Here's how the part is built. I have some questions about the finished solid (model axes, mm). Coordinates: 2 decimals unless noted, no trailing zeros. Write each loop counter-clockwise with the first axis right and the second up, starting at its lowest first coordinate (ties: lowest second). Pieces come first, ordered by that corner, then holes. Notation, with made-up numbers: (70, -27.5) - (123, -27.5) arc R15 ccw to (123, -12.5) - close; hole circle Ø5 at (59.25, 47). An arc over 180 degrees is marked (long way). Answer in a Markdown table with one row per item. Add a question column.
Item 1: If I drill on probe 1 along Z at (x, y) = (-12.5, 2.7) (3 decimals); probe 2 along Z at (x, y) = (24.6, 0.85) (3 decimals); probe 3 along Z at (x, y) = (-24.5, 1.9) (3 decimals), over which ranges is the centre line in solid material (lowest first)? Write a range as from..to.
Item 2: Imagine slicing it at A-A (x = 24.6). Please give me the cut outline in (y, z) (3 decimals).
Item 3: Imagine slicing it at C-C (x = 3.5). Please give me the cut outline in (y, z), plus the area to 3 significant figures.
Item 4: Imagine slicing it at D-D (z = 0). Please give me the cut outline in (x, y) (1 decimal).
Item 5: Imagine slicing it at B-B (z = 25.8). Please give me the cut outline in (x, y) (3 decimals), plus the area to 3 significant figures.
Autodesk Inventor part; units mm, degrees
ref_plane "YZ Plane" through (0, 0, 0) normal (1, 0, 0) x (0, 1, 0)
ref_plane "XZ Plane" through (0, 0, 0) normal (0, 1, 0) x (-1, 0, 0)
ref_plane "XY Plane" through (0, 0, 0) normal (0, 0, 1) x (1, 0, 0)
sketch "Boceto1" plane through (0, 0, 0) normal (0, 1, 0) x (-1, 0, 0)
  line L0 (-31.7268, 34.9358) -> (-31.7268, -34.7768)
  line L1 (-28.9268, -37.5768) -> (25.401, -37.5769)
  line L2 (28.2018, -34.7802) -> (28.2019, 34.9339)
  line L3 (25.4109, 37.7268) -> (-28.9358, 37.7268)
  line L4 (-29.925, -4.425) -> (-29.925, 4.575)
  line L5 (-29.925, 4.575) -> (-29.85, 4.575)
  line L6 (-29.85, 4.575) -> (-27.6, 4.575)
  line L7 (-27.6, 4.575) -> (-27.525, 4.575)
  line L8 (-27.525, 4.575) -> (-27.525, -4.425)
  line L9 (-27.525, -4.425) -> (-27.6, -4.425)
  line L10 (-27.6, -4.425) -> (-29.85, -4.425)
  line L11 (-29.85, -4.425) -> (-29.925, -4.425)
  line L12 (26.4, -4.425) -> (26.325, -4.425)
  line L13 (26.325, -4.425) -> (24.075, -4.425)
  line L14 (24.075, -4.425) -> (24, -4.425)
  line L15 (24, -4.425) -> (24, 4.575)
  line L16 (24, 4.575) -> (24.075, 4.575)
  line L17 (24.075, 4.575) -> (26.325, 4.575)
  line L18 (26.325, 4.575) -> (26.4, 4.575)
  line L19 (26.4, 4.575) -> (26.4, -4.425)
  line L20 (26.325, 26.925) -> (26.4, 26.925)
  line L21 (26.4, 26.925) -> (26.4, 17.925)
  line L22 (26.4, 17.925) -> (26.325, 17.925)
  line L23 (26.325, 17.925) -> (24.075, 17.925)
  line L24 (24.075, 17.925) -> (24, 17.925)
  line L25 (24, 17.925) -> (24, 26.925)
  line L26 (24, 26.925) -> (24.075, 26.925)
  line L27 (24.075, 26.925) -> (26.325, 26.925)
  line L28 (-19.1813, -35.775) -> (-19.1813, -35.7)
  line L29 (-19.1813, -35.7) -> (-19.1813, -33.45)
  line L30 (-19.1813, -33.45) -> (-19.1813, -33.375)
  line L31 (-19.1813, -33.375) -> (-10.1813, -33.375)
  line L32 (-10.1813, -33.375) -> (-10.1813, -33.45)
  line L33 (-10.1813, -33.45) -> (-10.1813, -35.7)
  line L34 (-10.1813, -35.7) -> (-10.1813, -35.775)
  line L35 (-10.1813, -35.775) -> (-19.1813, -35.775)
  line L36 (6.6562, 33.525) -> (6.6562, 33.6)
  line L37 (6.6562, 33.6) -> (6.6562, 35.85)
  line L38 (6.6562, 35.85) -> (6.6562, 35.925)
  line L39 (6.6562, 35.925) -> (15.6562, 35.925)
  line L40 (15.6562, 35.925) -> (15.6562, 35.85)
  line L41 (15.6562, 35.85) -> (15.6562, 33.6)
  line L42 (15.6562, 33.6) -> (15.6562, 33.525)
  line L43 (15.6562, 33.525) -> (6.6562, 33.525)
  line L44 (-19.1813, 33.525) -> (-19.1813, 33.6)
  line L45 (-19.1813, 33.6) -> (-19.1813, 35.85)
  line L46 (-19.1813, 35.85) -> (-19.1813, 35.925)
  line L47 (-19.1813, 35.925) -> (-10.1813, 35.925)
  line L48 (-10.1813, 35.925) -> (-10.1813, 35.85)
  line L49 (-10.1813, 35.85) -> (-10.1813, 33.6)
  line L50 (-10.1813, 33.6) -> (-10.1813, 33.525)
  line L51 (-10.1813, 33.525) -> (-19.1813, 33.525)
  line L52 (24.075, -17.775) -> (26.325, -17.775)
  line L53 (26.325, -17.775) -> (26.4, -17.775)
  line L54 (26.4, -17.775) -> (26.4, -26.775)
  line L55 (26.4, -26.775) -> (26.325, -26.775)
  line L56 (26.325, -26.775) -> (24.075, -26.775)
  line L57 (24.075, -26.775) -> (24, -26.775)
  line L58 (24, -26.775) -> (24, -17.775)
  line L59 (24, -17.775) -> (24.075, -17.775)
  line L60 (6.6562, -35.775) -> (6.6562, -35.7)
  line L61 (6.6562, -35.7) -> (6.6562, -33.45)
  line L62 (6.6562, -33.45) -> (6.6562, -33.375)
  line L63 (6.6562, -33.375) -> (15.6562, -33.375)
  line L64 (15.6562, -33.375) -> (15.6562, -33.45)
  line L65 (15.6562, -33.45) -> (15.6562, -35.7)
  line L66 (15.6562, -35.7) -> (15.6562, -35.775)
  line L67 (15.6562, -35.775) -> (6.6562, -35.775)
  line L68 (-27.6, -26.775) -> (-29.85, -26.775)
  line L69 (-29.85, -26.775) -> (-29.925, -26.775)
  line L70 (-29.925, -26.775) -> (-29.925, -17.775)
  line L71 (-29.925, -17.775) -> (-29.85, -17.775)
  line L72 (-29.85, -17.775) -> (-27.6, -17.775)
  line L73 (-27.6, -17.775) -> (-27.525, -17.775)
  line L74 (-27.525, -17.775) -> (-27.525, -26.775)
  line L75 (-27.525, -26.775) -> (-27.6, -26.775)
  line L76 (-27.525, 26.925) -> (-27.525, 17.925)
  line L77 (-27.525, 17.925) -> (-27.6, 17.925)
  line L78 (-27.6, 17.925) -> (-29.85, 17.925)
  line L79 (-29.85, 17.925) -> (-29.925, 17.925)
  line L80 (-29.925, 17.925) -> (-29.925, 26.925)
  line L81 (-29.925, 26.925) -> (-29.85, 26.925)
  line L82 (-29.85, 26.925) -> (-27.6, 26.925)
  line L83 (-27.6, 26.925) -> (-27.525, 26.925)
  line L84 (-2.25, -17.475) -> (2.25, -17.475)
  line L85 (2.25, -17.475) -> (2.25, -22.725)
  line L86 (2.25, -22.725) -> (-2.25, -22.725)
  line L87 (-2.25, -22.725) -> (-2.25, -17.475)
  circle A0 centre (-24.6, 25.8) radius 1.05
  circle A1 centre (21.075, 25.8) radius 1.05
  circle A2 centre (0, 0) radius 5.4375
  arc A3 (-31.7268, -34.7768) -> (-28.9268, -37.5768) centre (-28.9268, -34.7768) ccw
  arc A4 (-28.9358, 37.7268) -> (-31.7268, 34.9358) centre (-28.9358, 34.9358) ccw
  arc A5 (25.401, -37.5769) -> (28.2018, -34.7802) centre (25.4018, -34.7769) ccw
  arc A6 (28.2019, 34.9339) -> (25.4109, 37.7268) centre (25.4108, 34.9357) ccw
  circle A7 centre (-24.6, -24.075) radius 1.05
  circle A8 centre (21.075, -24.075) radius 1.05
  line L88 (15.6562, 35.925) -> (6.6562, 35.925)
  line L89 (6.6562, 35.925) -> (6.6562, 33.525)
  line L90 (6.6562, 33.525) -> (15.6562, 33.525)
  line L91 (15.6562, 33.525) -> (15.6562, 35.925)
  line L92 (26.4, 26.925) -> (24, 26.925)
  line L93 (24, 26.925) -> (24, 17.925)
  line L94 (24, 17.925) -> (26.4, 17.925)
  line L95 (26.4, 17.925) -> (26.4, 26.925)
  line L96 (26.4, 4.575) -> (24, 4.575)
  line L97 (24, 4.575) -> (24, -4.425)
  line L98 (24, -4.425) -> (26.4, -4.425)
  line L99 (26.4, -4.425) -> (26.4, 4.575)
  line L100 (26.4, -17.775) -> (24, -17.775)
  line L101 (24, -17.775) -> (24, -26.775)
  line L102 (24, -26.775) -> (26.4, -26.775)
  line L103 (26.4, -26.775) -> (26.4, -17.775)
  line L104 (15.6562, -33.375) -> (6.6562, -33.375)
  line L105 (6.6562, -33.375) -> (6.6562, -35.775)
  line L106 (6.6562, -35.775) -> (15.6562, -35.775)
  line L107 (15.6562, -35.775) -> (15.6562, -33.375)
  line L108 (-10.1813, -33.375) -> (-19.1813, -33.375)
  line L109 (-19.1813, -33.375) -> (-19.1813, -35.775)
  line L110 (-19.1813, -35.775) -> (-10.1813, -35.775)
  line L111 (-10.1813, -35.775) -> (-10.1813, -33.375)
  line L112 (-27.525, -26.775) -> (-29.925, -26.775)
  line L113 (-29.925, -26.775) -> (-29.925, -17.775)
  line L114 (-29.925, -17.775) -> (-27.525, -17.775)
  line L115 (-27.525, -17.775) -> (-27.525, -26.775)
  line L116 (-27.525, -4.425) -> (-29.925, -4.425)
  line L117 (-29.925, -4.425) -> (-29.925, 4.575)
  line L118 (-29.925, 4.575) -> (-27.525, 4.575)
  line L119 (-27.525, 4.575) -> (-27.525, -4.425)
  line L120 (-27.525, 17.925) -> (-29.925, 17.925)
  line L121 (-29.925, 17.925) -> (-29.925, 26.925)
  line L122 (-29.925, 26.925) -> (-27.525, 26.925)
  line L123 (-27.525, 26.925) -> (-27.525, 17.925)
  line L124 (-19.1813, 35.925) -> (-10.1813, 35.925)
  line L125 (-10.1813, 35.925) -> (-10.1813, 33.525)
  line L126 (-10.1813, 33.525) -> (-19.1813, 33.525)
  line L127 (-19.1813, 33.525) -> (-19.1813, 35.925)
  line L128 (2.25, -17.475) -> (-2.25, -17.475)
  line L129 (-2.25, -17.475) -> (-2.25, -22.725)
  line L130 (-2.25, -22.725) -> (2.25, -22.725)
  line L131 (2.25, -22.725) -> (2.25, -17.475)
extrude "Extrusión1" add sketch "Boceto1" along normal blind 3
properties part number "tapa2"
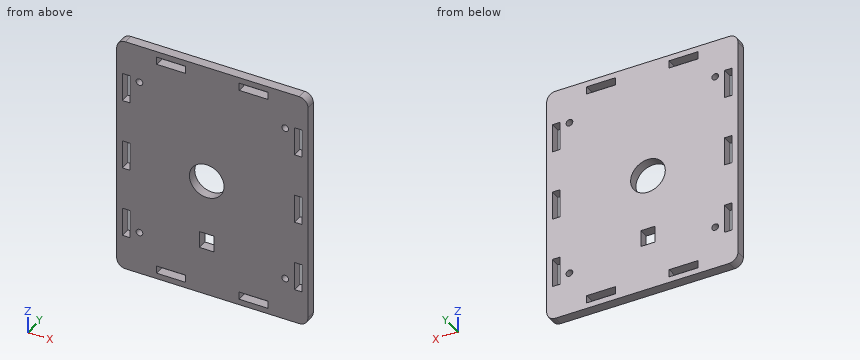
Here are the results:
| question | item | result |
|---|---|---|
| 1 | probe 1 | z = -37.577..-35.775, -33.375..33.525, 35.925..37.727 |
| 1 | probe 2 | z = -37.577..-25.125, -23.025..24.75, 26.85..37.727 |
| 1 | probe 3 | z = -37.577..-26.775, -17.775..-4.425, 4.575..17.925, 26.925..37.727 |
| 2 | outline | (0, -37.577) - (3, -37.577) - (3, -25.125) - (0, -25.125) - close; (0, -23.025) - (3, -23.025) - (3, 24.75) - (0, 24.75) - close; (0, 26.85) - (3, 26.85) - (3, 37.727) - (0, 37.727) - close |
| 3 | outline | (0, -37.58) - (3, -37.58) - (3, -4.16) - (0, -4.16) - close; (0, 4.16) - (3, 4.16) - (3, 37.73) - (0, 37.73) - close |
| 3 | area | 201 mm2 |
| 4 | outline | (-28.2, 0) - (-26.4, 0) - (-26.4, 3) - (-28.2, 3) - close; (-24, 0) - (-5.4, 0) - (-5.4, 3) - (-24, 3) - close; (5.4, 0) - (27.5, 0) - (27.5, 3) - (5.4, 3) - close; (29.9, 0) - (31.7, 0) - (31.7, 3) - (29.9, 3) - close |
| 5 | outline | (-28.202, 0) - (-26.4, 0) - (-26.4, 3) - (-28.202, 3) - close; (-24, 0) - (-22.125, 0) - (-22.125, 3) - (-24, 3) - close; (-20.025, 0) - (23.55, 0) - (23.55, 3) - (-20.025, 3) - close; (25.65, 0) - (27.525, 0) - (27.525, 3) - (25.65, 3) - close; (29.925, 0) - (31.727, 0) - (31.727, 3) - (29.925, 3) - close |
| 5 | area | 153 mm2 |
